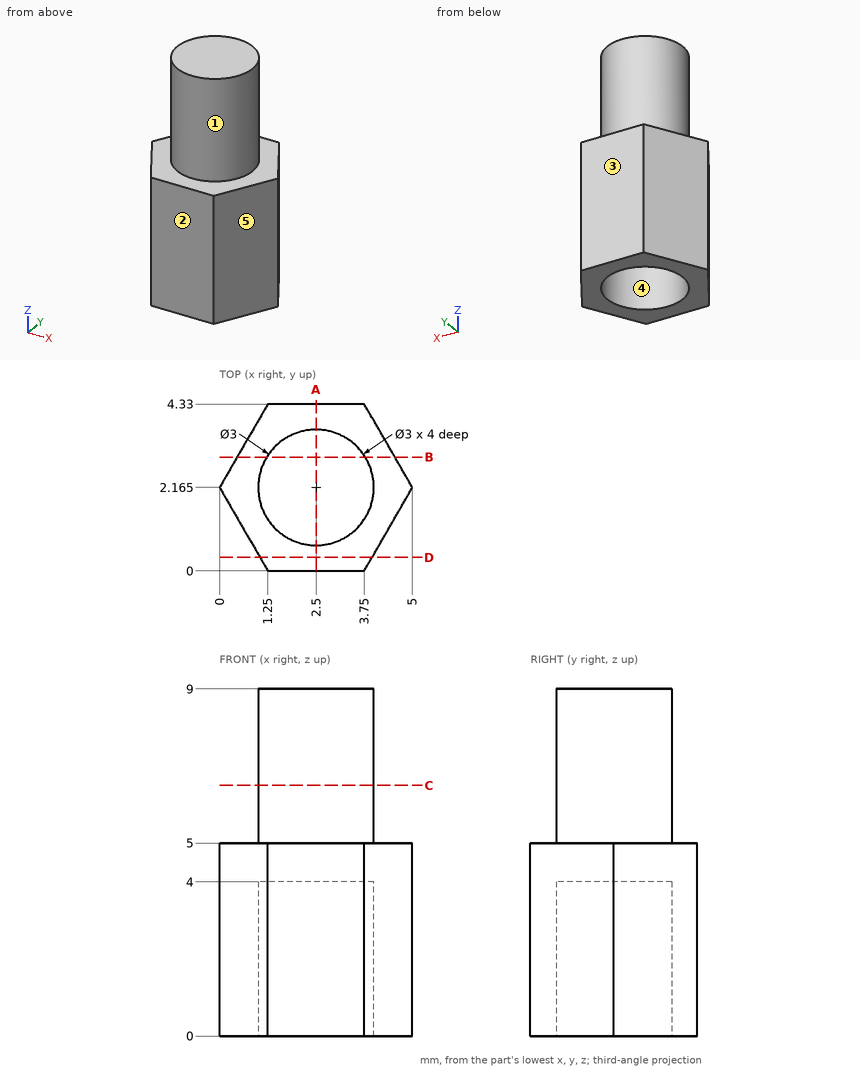
Can you work these out from the drawing? Everything is in mm from the part's minimum corner. A direction names the side the tool comes from. Round coordinates to 2 decimals unless told otherwise and drop trailing zeros. Order: outer loops, then holes, each group sorted by start corner. A loop starts at its lowest first (then second) coordinate and runs counter-clockwise, first axis right, second up. Notation, with made-up numbers: (59.5, 77) -> (94.5, 77) arc R9 cw to (94.5, 92) -> close; hole circle Ø9 at (15.5, 70). An arc over 180 degrees is marked (long way). Use CSV: the item, a comma, the result in double quotes.
1. I want a section at B-B on y = 2.95. List the corners of the cut face in (x, z) for me.
Recorded:
outline,"(0.45, 0) -> (1.22, 0) -> (1.22, 4) -> (3.78, 4) -> (3.78, 0) -> (4.55, 0) -> (4.55, 5) -> (3.78, 5) -> (3.78, 9) -> (1.22, 9) -> (1.22, 5) -> (0.45, 5) -> close"
2. Thinking about a two-plate mould opening in Y: for the marked faces 3, 4 and 5, which applies, pulls with the +Y half, pulls with the -Y half, needs draft (parallel to the pull), parting line crosses it, or undercut?
Recorded:
face 3,"pulls with the +Y half"
face 4,"undercut"
face 5,"pulls with the -Y half"
3. I want a section at A-A on x = 2.5. List the corners of the cut face in (y, z) for me (3 decimals).
Recorded:
outline,"(0, 0) -> (0.665, 0) -> (0.665, 4) -> (3.665, 4) -> (3.665, 0) -> (4.33, 0) -> (4.33, 5) -> (3.665, 5) -> (3.665, 9) -> (0.665, 9) -> (0.665, 5) -> (0, 5) -> close"
4. Which directions (+Z, -Z, +X, -X, +Y, -Y) give clear straight access to the entire face, cutting with the end or side of a thin tool? Please do the marked faces 1 and 2.
Recorded:
face 1,"+Z"
face 2,"+Z, -Z, +X, -X, -Y"
5. I want a section at C-C on z = 6.5. List the corners of the cut face in (x, y) for me (3 decimals).
Recorded:
outline,"circle Ø3 at (2.5, 2.165)"
6. I want a section at D-D on y = 0.35. List the corners of the cut face in (x, z) for me.
Recorded:
outline,"(1.05, 0) -> (3.95, 0) -> (3.95, 5) -> (1.05, 5) -> close"
7. I need wall thicknesses on line 1 along Y through (x, z) = (2.5, 2.35) (3 decimals); line 2 along Z through (x, y) = (2.9, 1.9); line 3 along X through (y, z) = (1.9, 1.75). Which ranges of each line are inside material? Lowest first, please.
Recorded:
line 1,"y = 0 to 0.665, 3.665 to 4.33"
line 2,"z = 4 to 9"
line 3,"x = 0.15 to 1.02, 3.98 to 4.85"
8. I'm going to push a flat-ended pin straight in: P1, Ø2.5, axis at x = 2.5, y = 2, coming from the -Z side. Where does the tip first touch, or does it pass through?
Recorded:
P1,"stops at z = 4"
